The listing builds one solid part. Answer for the finished solid, in the listing's coordinates (mm). Face numbers are marked on the shaded views. A direction names the side the tool comes from. Give positions to 0.01 mm unless a question says otherwise; leave off trailing zeros. Order: outer loops, then holes, each group sorted by start corner. A loop starts at its lowest first (then second) coordinate and runs counter-clockwise, first axis right, second up. Notation, with made-up numbers: (-34.75, 83) - (-0.75, 83) arc R25 cw to (-0.75, 112) - close; hole circle Ø3 at (6.5, 75.5). An arc over 180 degrees is marked (long way). Answer as a JSON object with one key per item and string values. Group by question number.
Q1. A cutting plane is placed at D-D, the plane y = 29. Count the separate pieces of the cut face and the enclosed holes in it, and give its area (3 significant figures).
Q2. Given pin 1 (19.5 mm diameter, centred on x = 5, y = 13.5, fed in from +Z); pin 2 (1 mm diameter, centred on y = 20, z = 11, fed in from -X); pin 3 (5 mm diameter, centred on x = 31, z = 21, fed in from -Y), each flat-ended and moving along its own axis, determine where each tip first touches the part or whether it passes through.
Q3. A cutting plane is placed at A-A, the plane y = 3. Give the vertices of the cut face in (x, z).
Q4. A cutting plane is placed at B-B, the plane x = 25. Give the vertices of the cut face in (y, z) (3 decimals), and give its area (3 significant figures).
Q5. A cutting plane is placed at C-C, the plane z = 19.05. Give the vertices of the cut face in (x, y).
Q6. The mould has two halves that part along Y. Classify the marked faces 6, 7 and 8: released by +Y, released by -Y, zero draft, split by the parting line, or undercut.
Q7. Consider line 1 (X direction, y = 32, z = 19.05); line 2 (X direction, y = 1.5, z = 7.25); line 3 (Y direction, x = -15.5, z = 4.5). Determine where each line is inside the solid, lowest interval first.
Q8. For the marked faces 1, 2, 3, 4 and 5, determine the directions among +Z, -Z, +X, -X, +Y, -Y from which every point of the face is accessible in a straight line to the end or side of a thin tool.
Autodesk Inventor part; units mm, degrees
ref_plane "YZ Plane" through (0, 0, 0) normal (1, 0, 0) x (0, 1, 0)
ref_plane "XZ Plane" through (0, 0, 0) normal (0, 1, 0) x (-1, 0, 0)
ref_plane "XY Plane" through (0, 0, 0) normal (0, 0, 1) x (1, 0, 0)
sketch "Sketch1" plane through (0, 0, 0) normal (0, 0, 1) x (1, 0, 0)
  line L0 (-19.1352, -8.5102) -> (-19.1352, 8.3898) construction
  line L1 (-16.8111, -6.1861) -> (-16.8111, 6.0657)
  line L2 (-21.4593, 6.0657) -> (-21.4593, -6.1861)
  arc A0 (-21.4593, -6.1861) -> (-16.8111, -6.1861) centre (-19.1352, -6.1861) ccw
  arc A1 (-16.8111, 6.0657) -> (-21.4593, 6.0657) centre (-19.1352, 6.0657) ccw
  line L3 (18.9648, -8.5102) -> (18.9648, 8.3898) construction
  line L4 (21.2889, -6.1861) -> (21.2889, 6.0657)
  line L5 (16.6407, 6.0657) -> (16.6407, -6.1861)
  arc A2 (16.6407, -6.1861) -> (21.2889, -6.1861) centre (18.9648, -6.1861) ccw
  arc A3 (21.2889, 6.0657) -> (16.6407, 6.0657) centre (18.9648, 6.0657) ccw
  line L6 (-19.1352, 8.3898) -> (18.9648, 8.3898)
  line L7 (18.9648, -8.5102) -> (-19.1352, -8.5102)
  line L8 (25.3148, 11.0523) -> (-25.4852, 11.0523)
  line L9 (-25.4852, 11.0523) -> (-25.4852, -11.1727)
  line L10 (-25.4852, -11.1727) -> (25.3148, -11.1727)
  line L11 (25.3148, -11.1727) -> (25.3148, 11.0523)
  line L12 (25.3148, 11.0523) -> (-25.4852, -11.1727) construction
  line L13 (-25.4852, 11.0523) -> (25.3148, -11.1727) construction
  point P0 (0, 0)
  point P1 (-0.0852, -0.0602)
  point P2 (-19.1352, -0.0602)
  point P3 (18.9648, -0.0602)
  dimension "d0" = 4.6482
  dimension "d1" = 4.6482
  dimension "d2" = 50.8
  dimension "d3" = 22.225
extrude "Extrusion1" add sketch "Sketch1" along normal blind 12.7 contours L1 A1 L6 A3 L5 A2 L7 A0 | L11 L10 L9 L8
sketch "Sketch2" plane through (-25.4852, 11.0523, 0) normal (0, 1, 0) x (1, 0, 0)
  line L0 (0, 0) -> (50.8, 0)
  line L1 (0, 0) -> (12.7, 0)
  line L2 (12.7, 0) -> (12.7, -12.7)
  line L3 (12.7, -12.7) -> (0, -12.7)
  line L4 (0, -12.7) -> (0, 0)
  line L5 (50.8073, 0) -> (38.1073, 0)
  line L6 (38.1073, 0) -> (38.1073, -12.7)
  line L7 (38.1073, -12.7) -> (50.8073, -12.7)
  line L8 (50.8, 0) -> (50.8, -12.7)
  line L9 (50.8, 0) -> (50.8, -12.7)
  line L10 (50.8, -12.7) -> (50.8, 0)
  line L11 (50.8, 0) -> (38.1073, 0)
  point P0 (25.4852, 0)
  dimension "d7" = 12.7
  dimension "d8" = 12.7
  dimension "d9" = 12.7
  dimension "d10" = 12.7
extrude "Extrusion2" add sketch "Sketch2" along normal blind 22.3933
chamfer "Chamfer1" distance 3.9688 distance2 5.5563 1 edges at (12.6221, 22.2489, 12.7) measured on face at (12.6221, 18.5167, 4.2333)
chamfer "Chamfer2" distance 4.7625 distance2 7.9375 1 edges at (-12.7852, 22.2489, 0) measured on face at (-12.7852, 18.5167, 8.4667)
sketch "Sketch3" plane through (-25.4852, 33.4456, 0) normal (0, 1, 0) x (1, 0, 0)
  line L0 (0, 0) -> (6.319, 0)
  line L1 (38.1073, 0) -> (4.7625, 0)
  line L2 (6.319, -0.6519) -> (0, -0.6519)
  line L3 (0, 0) -> (0, -12.7)
  line L4 (0, 0) -> (0, -0.6519)
  line L5 (6.319, 0) -> (6.319, -0.6519)
  point P0 (25.4852, 0)
extrude "Extrusion3" cut sketch "Sketch3" against normal up to surface (22.3933 mm away)
fillet "Fillet2" radius 3.175 2 edges at (-19.6363, 22.2489, 0.6519) (-25.4852, 22.2489, 0.6519)
sketch "Sketch4" plane through (0, 0, 12.7) normal (0, 0, 1) x (1, 0, 0)
  line L0 (-12.7852, 11.0523) -> (-18.8822, 11.0523)
  line L1 (-12.7852, 11.0523) -> (-12.7852, 26.6987)
  line L2 (-12.7852, 33.4456) -> (-12.7852, 11.0523)
  line L3 (-12.7852, 11.0523) -> (25.3148, 11.0523)
  line L4 (25.3148, -11.1727) -> (25.3148, 33.4456)
  line L5 (25.3148, 11.0523) -> (25.3148, 26.6987)
  line L6 (12.6221, 33.4456) -> (12.6221, 11.0523)
  line L7 (-25.4852, -11.1727) -> (-25.4852, 33.4456)
  line L8 (25.3148, 26.6987) -> (12.6221, 26.6987)
  line L9 (12.6221, 26.6987) -> (12.6221, 36.2237)
  line L10 (25.3148, 36.2237) -> (25.3148, 26.6987)
  line L11 (-12.7852, 26.6987) -> (-25.4852, 26.6987)
  line L12 (-25.4852, 26.6987) -> (-25.4852, 36.2237)
  line L13 (-12.7852, 36.2237) -> (-12.7852, 26.6987)
  line L14 (18.1783, 33.4456) -> (12.6221, 33.4456)
  line L15 (25.3148, 33.4456) -> (12.6221, 33.4456)
  line L16 (-12.7852, 36.2237) -> (-12.7852, 33.4456)
  line L17 (-25.4852, 33.4456) -> (-12.7852, 33.4456)
  line L18 (-12.7852, 33.4456) -> (-25.4852, 33.4456)
  line L19 (-25.4852, 33.4456) -> (-25.4852, 36.2237)
  line L20 (12.6221, 33.4456) -> (12.6221, 26.6987)
  line L21 (25.3148, 26.6987) -> (25.3148, 33.4456)
  line L22 (-12.7852, 26.6987) -> (-12.7852, 33.4456)
  line L23 (-25.4852, 26.6987) -> (-25.4852, 33.4456)
  point P0 (0, 0)
  dimension "d22" = 15.6464
extrude "Extrusion4" add sketch "Sketch4" along normal blind 12.7 contours L2 L11 L7 L17 | L6 L14 L15 L4 L8
extrude "Extrusion5" add sketch "Sketch4" against normal blind 4.2333 contours L6 L14 L15 L4 L8
sketch "Sketch5" plane through (-25.4852, 33.4456, 0) normal (0, 1, 0) x (1, 0, 0)
  line L0 (50.8, -25.4) -> (38.1073, -25.4)
  line L1 (12.7, -25.4) -> (0, -25.4)
  line L2 (44.4537, -25.4) -> (44.4537, -19.05)
  line L3 (6.35, -25.4) -> (6.35, -19.05)
  circle A0 centre (6.35, -19.05) radius 2.3241
  circle A1 centre (44.4537, -19.05) radius 2.3241
  point P0 (25.4852, 0)
  dimension "d27" = 6.35
  dimension "d28" = 6.35
  dimension "d29" = 4.6482
  dimension "d30" = 4.6482
extrude "Extrusion6" cut sketch "Sketch5" against normal through all
sketch "Sketch6" plane through (-12.7852, 11.0523, 12.7) normal (1, 0, 0) x (0, 0, -1)
  line L0 (-12.7, 15.6464) -> (-12.7, 22.3933)
  line L1 (0, 15.6464) -> (-12.7, 15.6464)
  line L2 (-12.7, 15.6464) -> (-12.7, 22.3933)
  line L3 (-12.7, 22.3933) -> (0, 22.3933)
  line L4 (0, 22.3933) -> (0, 15.6464)
  line L5 (0, 15.6464) -> (-12.7, 15.6464)
  point P0 (12.7, -11.0523)
extrude "Extrusion7" [suppressed]
sketch "Sketch7" plane through (18.1783, 26.6987, 12.7) normal (0, -1, 0) x (1, 0, 0)
  circle A0 centre (-37.3136, 6.35) radius 2.3241
  circle A1 centre (0.7901, 6.35) radius 2.3241
  line L0 (-37.3136, 6.35) -> (-24.6136, 6.35)
  line L1 (-24.6136, 6.35) -> (-11.9136, 6.35)
  line L2 (-26.798, 4.1656) -> (-22.4292, 4.1656)
  line L3 (-22.4292, 4.1656) -> (-22.4292, 8.5344)
  line L4 (-22.4292, 8.5344) -> (-26.798, 8.5344)
  line L5 (-26.798, 8.5344) -> (-26.798, 4.1656)
  line L6 (-26.798, 4.1656) -> (-22.4292, 8.5344) construction
  line L7 (-22.4292, 4.1656) -> (-26.798, 8.5344) construction
  line L8 (-9.7292, 8.5344) -> (-14.098, 8.5344)
  line L9 (-9.7292, 4.1656) -> (-9.7292, 8.5344)
  line L10 (-14.098, 4.1656) -> (-9.7292, 4.1656)
  line L11 (-14.098, 8.5344) -> (-14.098, 4.1656)
  point P0 (-18.1783, -12.7)
  dimension "d35" = 12.7
  dimension "d36" = 12.7
  dimension "d37" = 4.3688
  dimension "d38" = 4.3688
  dimension "d41" = 12.7
extrude "Extrusion8" [suppressed]
fillet "Fillet3" [suppressed]
sketch "Sketch8" plane through (-25.4852, 11.0523, 0) normal (0, 1, 0) x (1, 0, 0)
  line L0 (38.1073, 0) -> (0, 0)
  line L1 (0, 0) -> (14.6548, 0)
  line L2 (14.6548, 0) -> (14.6548, -26.951)
  line L3 (14.6548, -26.951) -> (0, -26.951)
  line L4 (0, -26.951) -> (0, 0)
  point P0 (25.4852, 0)
  point P1 (14.6548, 0)
extrude "Extrusion9" cut sketch "Sketch8" along normal blind 25.4
sketch "Sketch9" plane through (25.3148, -11.1727, 12.7) normal (1, 0, 0) x (0, 0, -1)
  line L0 (0, 0) -> (0, 37.8714)
  line L1 (12.7, 0) -> (0, 0)
  line L2 (12.7, 0) -> (12.7, 44.6183)
  line L3 (12.7, 44.6183) -> (-12.7, 44.6183)
  line L4 (-12.7, 37.8714) -> (-12.7, 44.6183)
  line L5 (0, 37.8714) -> (-12.7, 37.8714)
  point P0 (12.7, 11.1727)
extrude "Extrusion10" add sketch "Sketch9" along normal blind 12.7
sketch "Sketch10" plane through (-25.4852, 33.4456, 0) normal (0, 1, 0) x (1, 0, 0)
  circle A0 centre (44.4537, -19.05) radius 2.3241
  line L0 (44.4537, -19.05) -> (57.1537, -19.05)
  circle A1 centre (57.1537, -19.05) radius 2.3241
  point P0 (25.4852, 0)
  dimension "d58" = 12.7
  dimension "d59" = 4.6482
extrude "Extrusion11" cut sketch "Sketch10" against normal blind 12.7 contours A1
fillet "Fillet9" radius 3.175 2 edges at (12.6221, 30.0721, 25.4) (38.0148, 30.0721, 25.4)
fillet "Fillet10" radius 6.35 3 edges at (-25.4852, 11.0523, 6.35) (-25.4852, -11.1727, 6.35) (38.0148, -11.1727, 6.35)
sketch "Sketch11" plane through (-25.4852, 33.4456, 0) normal (0, 1, 0) x (1, 0, 0)
  arc A0 (60.325, -25.4) -> (63.5, -22.225) centre (60.325, -22.225) ccw
  line L0 (63.5, 0) -> (63.5, -22.225)
  line L1 (38.1073, 0) -> (63.5, 0)
  line L2 (38.1073, 0) -> (38.1073, -22.225)
  arc A1 (38.1073, -22.225) -> (41.2823, -25.4) centre (41.2823, -22.225) ccw
  line L3 (41.2823, -25.4) -> (60.325, -25.4)
  circle A2 centre (57.1537, -19.05) radius 2.3241
  circle A3 centre (44.4537, -19.05) radius 2.3241
  point P0 (25.4852, 0)
extrude "Extrusion12" add sketch "Sketch11" along normal blind 1.5875
sketch "Sketch12" plane through (18.1783, 26.6987, 12.7) normal (0, -1, 0) x (1, 0, 0)
  circle A0 centre (13.4901, 6.35) radius 2.3241
  circle A1 centre (0.7901, 6.35) radius 2.3241
  arc A2 (19.8364, 9.525) -> (16.6614, 12.7) centre (16.6614, 9.525) ccw
  line L0 (-2.3813, 12.7) -> (16.6614, 12.7)
  arc A3 (-2.3813, 12.7) -> (-5.5563, 9.525) centre (-2.3813, 9.525) ccw
  line L1 (-5.5563, -3.9688) -> (-5.5563, 9.525)
  line L2 (0, 0) -> (-5.5563, -3.9688)
  line L3 (19.8364, 0) -> (0, 0)
  line L4 (19.8364, 9.525) -> (19.8364, 0)
  point P0 (-18.1783, -12.7)
extrude "Extrusion13" cut sketch "Sketch12" against normal blind 1.5875
fillet "Fillet12" radius 3.175 1 edges at (25.3184, 35.0331, 0)
properties part number "Optical Mount"
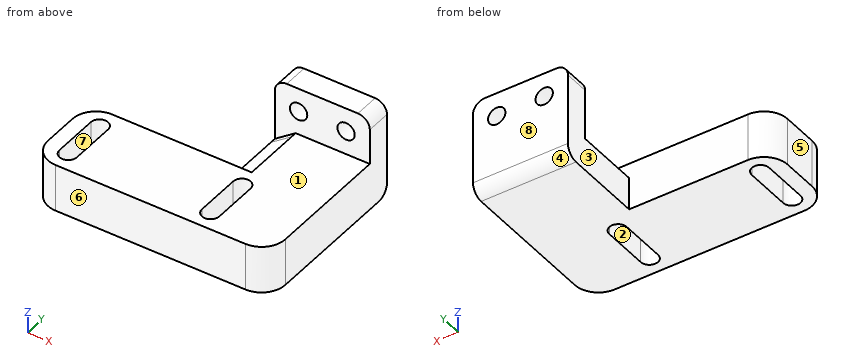
Reply:
{
 "1": {"separate pieces": "1", "enclosed holes": "2", "area": "607 mm^2"},
 "2": {"pin 1": "stops at z = 12.7", "pin 2": "stops at x = 15.1", "pin 3": "stops at y = 28.29"},
 "3": {"outline": "(-25.49, 0) - (-21.46, 0) - (-21.46, 12.7) - (-25.49, 12.7) - close; (-16.81, 0) - (16.64, 0) - (16.64, 12.7) - (-16.81, 12.7) - close; (21.29, 0) - (38.01, 0) - (38.01, 12.7) - (21.29, 12.7) - close"},
 "4": {"outline": "(-11.173, 0) - (31.858, 0) arc R3.175 ccw to (35.033, 3.175) - (35.033, 25.4) - (28.286, 25.4) - (28.286, 12.7) - (-11.173, 12.7) - close", "area": "670 mm^2"},
 "5": {"outline": "(12.62, 28.29) - (16.64, 28.29) - (16.64, 35.03) - (12.62, 35.03) - close; (21.29, 28.29) - (29.34, 28.29) - (29.34, 35.03) - (21.29, 35.03) - close; (33.99, 28.29) - (38.01, 28.29) - (38.01, 35.03) - (33.99, 35.03) - close"},
 "6": {"face 6": "released by -Y", "face 7": "undercut", "face 8": "released by +Y"},
 "7": {"line 1": "x = 12.62 to 16.64, 21.29 to 29.34, 33.99 to 38.01", "line 2": "x = -25.49 to -21.46, -16.81 to 16.64, 21.29 to 38.01", "line 3": "y = -11.17 to 11.05"},
 "8": {"face 1": "+Z, +X, -X, -Y", "face 2": "+Z, -Z", "face 3": "+Z, -Z, -X, +Y", "face 4": "-Z, +X, -X, +Y", "face 5": "+Z, -Z, -X, +Y, -Y"}
}
